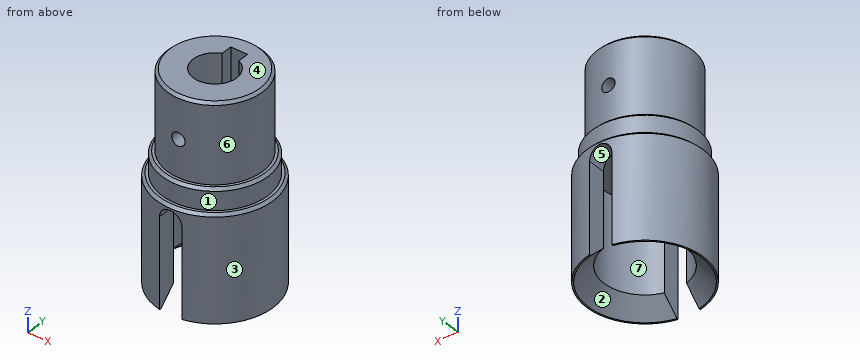
from build123d import *

# Parameters (mm, degrees)
SKETCH_1_R           = 11
EXTRUDE_1_DEPTH      = 29
SKETCH_2_OUTSIDE_W   = 32.506
SKETCH_2_OUTSIDE_H   = 32.506
SKETCH_2_OUTSIDE_R   = 10
CUT_EXTRUDE_1_DEPTH  = 9
SKETCH_3_R           = 7.7
CUT_EXTRUDE_2_DEPTH  = 20
SKETCH_4_R           = 2.1
CUT_EXTRUDE_3_DEPTH  = 25
CHAMFER_1_SIZE       = 3
EXTRUDE_START        = 10
SKETCH_5_R           = 10
EXTRUDE_2_DEPTH      = 10
SKETCH_6_R           = 4
CUT_EXTRUDE_5_DEPTH  = 19
SKETCH_8_OUTSIDE_W   = 33.978
SKETCH_8_OUTSIDE_H   = 33.978
SKETCH_8_OUTSIDE_R   = 9
CUT_EXTRUDE_7_DEPTH  = 15
SKETCH_9_R           = 1.25
CUT_EXTRUDE_8_DEPTH  = 25
CHAMFER_3_SIZE       = 0.5
CUT_EXTRUDE_9_DEPTH  = 19
CUT_EXTRUDE_10_DEPTH = 19


with BuildPart() as part:
    # 草图1 → 凸台-拉伸1 (new body)
    with BuildSketch(Plane.XY):
        with Locations(Location((0, 0, 0), (0, 0, 180))):
            Circle(SKETCH_1_R)
    extrude(amount=EXTRUDE_1_DEPTH)

    # 草图2 outside → 切除-拉伸1 (cut)
    with BuildSketch(Plane.XY.offset(29)):
        Rectangle(SKETCH_2_OUTSIDE_W, SKETCH_2_OUTSIDE_H)
        Circle(SKETCH_2_OUTSIDE_R, mode=Mode.SUBTRACT)
    extrude(amount=-CUT_EXTRUDE_1_DEPTH, mode=Mode.SUBTRACT)

    # 草图3 → 切除-拉伸2 (cut)
    with BuildSketch(Plane(origin=(0, 0, 0), x_dir=(-1, 0, 0), z_dir=(0, 0, -1))):
        Circle(SKETCH_3_R)
    extrude(amount=-CUT_EXTRUDE_2_DEPTH, mode=Mode.SUBTRACT)

    # 草图4 → 切除-拉伸3 (cut, symmetric)
    with BuildSketch(Plane(origin=(0, 0, 0), x_dir=(1, 0, 0), z_dir=(0, 1, 0))):
        with BuildLine():
            Line((-2.1, 0), (-2.1, -17))
            ThreePointArc((-2.1, -17), (0, -14.9), (2.1, -17))
            Line((2.1, -17), (2.1, 0))
            Line((2.1, 0), (-2.1, 0))
        make_face()
        with Locations((0, -17)):
            Circle(SKETCH_4_R)
    extrude(amount=CUT_EXTRUDE_3_DEPTH, both=True, mode=Mode.SUBTRACT)

    # 倒角1
    chamfer_1_edges = [part.edges().sort_by_distance(p)[0] for p in [
        (7.7, 0, 0),
        (-6.142475071, -4.643274706, 0),
    ]]
    chamfer(chamfer_1_edges, length=CHAMFER_1_SIZE)

    # 草图5 → 凸台-拉伸2 (add)
    with BuildSketch(Plane.XY.offset(29).offset(EXTRUDE_START)):
        Circle(SKETCH_5_R)
    extrude(amount=-EXTRUDE_2_DEPTH)

    # 草图6 → 切除-拉伸5 (cut)
    with BuildSketch(Plane.XY.offset(39)):
        Circle(SKETCH_6_R)
    extrude(amount=-CUT_EXTRUDE_5_DEPTH, mode=Mode.SUBTRACT)

    # 草图8 outside → 切除-拉伸7 (cut)
    with BuildSketch(Plane.XY.offset(39)):
        Rectangle(SKETCH_8_OUTSIDE_W, SKETCH_8_OUTSIDE_H)
        Circle(SKETCH_8_OUTSIDE_R, mode=Mode.SUBTRACT)
    extrude(amount=-CUT_EXTRUDE_7_DEPTH, mode=Mode.SUBTRACT)

    # 草图9 → 切除-拉伸8 (cut, symmetric)
    with BuildSketch(Plane(origin=(0, 0, 0), x_dir=(1, 0, 0), z_dir=(0, 1, 0))):
        with Locations(Location((0, -31, 0), (0, 0, 270))):
            Circle(SKETCH_9_R)
    extrude(amount=CUT_EXTRUDE_8_DEPTH, both=True, mode=Mode.SUBTRACT)

    # 倒角3
    chamfer_3_edges = [part.edges().sort_by_distance(p)[0] for p in [
        (-10, 0, 24),
        (-9, 0, 39),
        (11, 0, 20),
    ]]
    chamfer(chamfer_3_edges, length=CHAMFER_3_SIZE)

    # 草图10 → 切除-拉伸9 (cut)
    with BuildSketch(Plane.XY.offset(39)):
        with BuildLine():
            Line((0, 5.8), (0, 4))
            ThreePointArc((0, 4), (0.76406905, 3.92634671), (1.5, 3.708099244))
            Line((1.5, 3.708099244), (1.5, 5.8))
            Line((1.5, 5.8), (0, 5.8))
        make_face()
        with BuildLine():
            ThreePointArc((-1.5, 3.708099244), (-0.76406905, 3.92634671), (0, 4))
            Line((0, 4), (0, 5.8))
            Line((0, 5.8), (-1.5, 5.8))
            Line((-1.5, 5.8), (-1.5, 3.708099244))
        make_face()
    extrude(amount=-CUT_EXTRUDE_9_DEPTH, mode=Mode.SUBTRACT)

    # 草图11 → 切除-拉伸10 (cut)
    with BuildSketch(Plane.XY.offset(39)):
        with BuildLine():
            Line((1.6, 3.774917218), (1.6, 5.9))
            Line((1.6, 5.9), (-1.6, 5.9))
            Line((-1.6, 5.9), (-1.6, 3.774917218))
            ThreePointArc((-1.6, 3.774917218), (0, -4.1), (1.6, 3.774917218))
        make_face()
    extrude(amount=-CUT_EXTRUDE_10_DEPTH, mode=Mode.SUBTRACT)


solid = part.part
Work out the finished part from the listing and answer in its coordinate system (mm). Face numbers are marked on the shaded views. A direction names the side the tool comes from. Coordinates: 2 decimals unless noted, no trailing zeros. Write each loop counter-clockwise with the first axis right and the second up, starting at its lowest first coordinate (ties: lowest second). Pieces come first, ordered by that corner, then holes. Notation, with made-up numbers: M -10,16.25 L 23,16.25 A15 ccw 23,33.25 Z; hole C -9,-12.5 d5. An arc over 180 degrees is marked long. Write item = value, one per line.
1. For the marked faces 1, 2 and 3, determine the directions among +Z, -Z, +X, -X, +Y, -Y from which every point of the face is accessible in a straight line to the end or side of a thin tool.
Solution:
face_1 = +Z
face_2 = -Z
face_3 = +Z, -Z
2. The part is cut by section D-D (z = 37). Determine the outline of the cut face in (x, y), then the cut area to 3 significant figures.
Solution:
outline = C 0,0 d18; hole M -1.6,3.77 A4.1 ccw long 1.6,3.77 L 1.6,5.9 L -1.6,5.9 Z
area = 196 mm2
3. The part is cut by section B-B (y = 0). Determine the outline of the cut face in (x, z).
Solution:
outline = M -11,0 L -10.7,0 L -7.7,3 L -7.7,20 L -4.1,20 L -4.1,39 L -8.5,39 L -9,38.5 L -9,24 L -9.5,24 L -10,23.5 L -10,20 L -10.5,20 L -11,19.5 Z; M 4.1,20 L 7.7,20 L 7.7,3 L 10.7,0 L 11,0 L 11,19.5 L 10.5,20 L 10,20 L 10,23.5 L 9.5,24 L 9,24 L 9,38.5 L 8.5,39 L 4.1,39 Z
4. The part is cut by section C-C (z = 12.5). Determine the outline of the cut face in (x, y).
Solution:
outline = M -2.1,-10.8 L -2.1,-7.41 A7.7 cw -2.1,7.41 L -2.1,10.8 A11 ccw Z; M 2.1,-10.8 A11 ccw 2.1,10.8 L 2.1,7.41 A7.7 cw 2.1,-7.41 Z
5. The part is cut by section A-A (x = 0). State how many separate pieces and enclosed holes the cut face has, then the cut area to 3 significant figures.
Solution:
separate_pieces = 4
enclosed_holes = 0
area = 145 mm2
6. Determine the mould class of the marked faces 4, 5, 6 and 7 for opening direction X: released by +X, released by -X, zero draft, split by the parting line, or undercut.
Solution:
face_4 = zero draft
face_5 = undercut
face_6 = split by the parting line
face_7 = undercut
7. Flat-ended cylindrical pins translate along their axes: pin 1 (2.5 mm diameter, centred on y = 5.5, z = 27.5, fed in from -X); pin 2 (6 mm diameter, centred on x = -8.5, y = -8, fed in from +Z); pin 3 (2.5 mm diameter, centred on y = 9, z = 11, fed in from +X). Find the tip coordinate at first contact, or state that the pin passes through.
Solution:
pin_1 = -7.93
pin_2 = 38.83
pin_3 = 7.81
8. Straight lines are drawn through the part: line 1 (Z direction, x = 0, y = -5.15); line 2 (Y direction, x = 0, z = 36.5); line 3 (Z direction, x = 5.25, y = 0.5). For each, find the intervals that lie inside material, in ascending order. Write a range as from..to.
Solution:
line_1 = 20..29.75, 32.25..39
line_2 = -9..-4.1, 5.9..9
line_3 = 20..39
